from build123d import *

# Parameters (mm, degrees)
F1_DEPTH = 150


with BuildPart() as f1:
    # F0 (on Front) → F1 (new body)
    with BuildSketch(Plane.XZ):
        with BuildLine():
            ThreePointArc((100, 202.087122), (84.900082, 249.700459), (58.472668, 292.087122))
            ThreePointArc((58.472668, 292.087122), (29.502824, 298.012806), (0, 300))
            ThreePointArc((0, 300), (-29.502824, 298.012806), (-58.472668, 292.087122))
            ThreePointArc((-58.472668, 292.087122), (-84.900082, 249.700459), (-100, 202.087122))
            ThreePointArc((-100, 202.087122), (-57.971121, 122.095615), (-50, 32.087122))
            ThreePointArc((-50, 32.087122), (-29.705148, 8.711728), (0, 0))
            ThreePointArc((0, 0), (29.705148, 8.711728), (50, 32.087122))
            ThreePointArc((50, 32.087122), (57.971121, 122.095615), (100, 202.087122))
        make_face()
    extrude(amount=F1_DEPTH)


solid = f1.part
The listing builds one solid part. Answer for the finished solid, in the listing's coordinates (mm). Give positions to 0.01 mm unless a question says otherwise; leave off trailing zeros. Write each loop counter-clockwise with the first axis right and the second up, starting at its lowest first coordinate (ties: lowest second). Pieces come first, ordered by that corner, then holes. Notation, with made-up numbers: (-27.5, -21) -> (12.5, -21) arc R20 cw to (12.5, -10) -> close; hole circle Ø3 at (39, 62). An arc over 180 degrees is marked (long way). One line per question, with ' | ' between items. Start each with the question number.
1. For a pull along Z with two mould halves and no side action, classify faces 1 (the cylindrical face through (-58.334, -73.95, 123.316)), 2 (the cylindrical face through (-84.605, -73.95, 250.337)), 3 (the flat face through (-1, 0, 152)) as pulls with the +Z half, pulls with the -Z half, needs draft (parallel to the pull), parting line crosses it, or undercut.
2. Find the intervals of material crossed by probe 1 along Z at (x, y) = (23, -108); probe 2 along X at (y, z) = (-14.5, 127.5); probe 3 along X at (y, z) = (-90, 104), in increasing order.
3. Section C-C (x = 64.5) is taken. Determine the outline of the cut face in (y, z), plus the area to 3 significant figures.
4. Given pin 1 Ø10 at (y, z) = (-34.5, 135.5) entering from -X; pin 2 Ø8 at (y, z) = (-53, 107) entering from -X; pin 3 Ø10 at (x, y) = (-46, -40.5) entering from -Z, each flat-ended and moving along its own axis, determine where each tip first touches the part or whether it passes through.
5. Section B-B (z = 260) is taken. Determine the outline of the cut face in (x, y).
6. Section A-A (y = -57) is taken. Determine the outline of the cut face in (x, z), plus the area to 3 significant figures.
Response values:
1) face 1: undercut | face 2: pulls with the +Z half | face 3: needs draft
2) probe 1: 5.04 to 298.79 | probe 2: -59.63 to 59.63 | probe 3: -53.44 to 53.44
3) outline: (-150, 141.16) -> (0, 141.16) -> (0, 284.29) -> (-150, 284.29) -> close | area: 21,500 mm2
4) pin 1: x = -64.24 | pin 2: x = -55.01 | pin 3: z = 18.34
5) outline: (-79.78, -150) -> (79.78, -150) -> (79.78, 0) -> (-79.78, 0) -> close
6) outline: (-100, 202.09) arc R230 cw to (-50, 32.09) arc R55 ccw to (0, 0) arc R55 ccw to (50, 32.09) arc R230 cw to (100, 202.09) arc R200 ccw to (58.47, 292.09) arc R220 ccw to (0, 300) arc R220 ccw to (-58.47, 292.09) arc R200 ccw to start | area: 39,300 mm2
